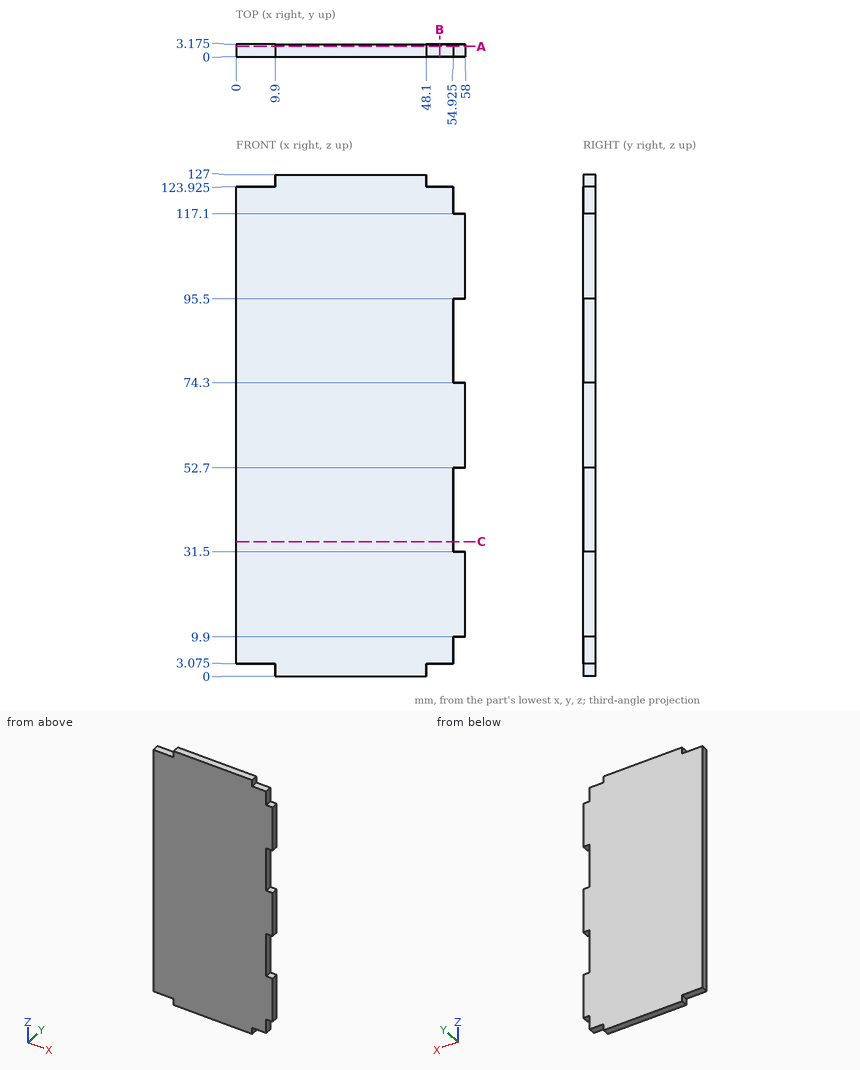
Job drawing, mm, ordinate dimensions from the low corner. One solid piece. Give positions to 0.01 mm unless a question says otherwise; leave off trailing zeros. Order: outer loops, then holes, each group sorted by start corner. A loop starts at its lowest first (then second) coordinate and runs counter-clockwise, first axis right, second up. Notation, with made-up numbers: (73, 83.5) - (79, 83.5) arc R14 ccw to (79, 105.5) - close; hole circle Ø10 at (40, -37). An arc over 180 degrees is marked (long way). Answer in a Markdown table with one row per item.
1. Saw through at C-C, the plane z = 34. Give the cut face in (x, y) (3 decimals), plus the area to 3 significant figures.
Data:
| item | result |
|---|---|
| outline | (0, 0) - (54.925, 0) - (54.925, 3.175) - (0, 3.175) - close |
| area | 174 mm² |
2. Probe probe 1 along Z at (x, y) = (49, 2.4) (3 decimals); probe 2 along X at (y, z) = (0.6, 94.5) (3 decimals). List the from-to ranges inside material, lowest first. Write a range as [from, to].
Data:
| item | result |
|---|---|
| probe 1 | z = [3.075, 123.925] |
| probe 2 | x = [0, 54.925] |
3. Saw through at B-B, the plane x = 51.5. Give the cut face in (y, z) (3 decimals), plus the area to 3 significant figures.
Data:
| item | result |
|---|---|
| outline | (0, 3.075) - (3.175, 3.075) - (3.175, 123.925) - (0, 123.925) - close |
| area | 384 mm² |
4. Saw through at A-A, the plane y = 2.6. Give the cut face in (x, z) (3 decimals).
Data:
| item | result |
|---|---|
| outline | (0, 3.075) - (9.9, 3.075) - (9.9, 0) - (48.1, 0) - (48.1, 3.075) - (54.925, 3.075) - (54.925, 9.9) - (58, 9.9) - (58, 31.5) - (54.925, 31.5) - (54.925, 52.7) - (58, 52.7) - (58, 74.3) - (54.925, 74.3) - (54.925, 95.5) - (58, 95.5) - (58, 117.1) - (54.925, 117.1) - (54.925, 123.925) - (48.1, 123.925) - (48.1, 127) - (9.9, 127) - (9.9, 123.925) - (0, 123.925) - close |
5. Flat gauge pins, fed straight in: pin 1 (1 mm diameter, centred on y = 2, z = 81, fed in from +X) (3 decimals); pin 2 (0.9 mm diameter, centred on x = 57, y = 1, fed in from +Z); pin 3 (1.5 mm diameter, centred on y = 2, z = 1.5, fed in from +X). Where does each tip first touch, or does it go through?
Data:
| item | result |
|---|---|
| pin 1 | stops at x = 54.925 |
| pin 2 | stops at z = 117.1 |
| pin 3 | stops at x = 48.1 |
